```python
from build123d import *
from OCP.BRepFilletAPI import BRepFilletAPI_MakeChamfer

# Parameters (mm, degrees)
SKETCH1_R           = 6.35
BOSS_EXTRUDE1_DEPTH = 450
SKETCH2_W           = 200
SKETCH2_H           = 200
BOSS_EXTRUDE2_DEPTH = 10
CHAMFER1_SIZE       = 10
CHAMFER1_SIZE_2     = 4.663076582
FILLET1_R           = 3


# Some blends are built 0.0001 mm under size
with BuildPart() as part:
    # Sketch1 → Boss-Extrude1 (new body)
    with BuildSketch(Plane(origin=(0, 0, 0), x_dir=(1, 0, 0), z_dir=(0, 1, 0))):
        with Locations(Location((0, 0, 0), (0, 0, 270))):
            Circle(SKETCH1_R)
    extrude(amount=BOSS_EXTRUDE1_DEPTH)

    # Sketch2 → Boss-Extrude2 (add)
    with BuildSketch(Plane(origin=(0, 0, 0), x_dir=(1, 0, 0), z_dir=(0, 1, 0))):
        with Locations((0, -70)):
            Rectangle(SKETCH2_W, SKETCH2_H)
    extrude(amount=BOSS_EXTRUDE2_DEPTH)

    # Chamfer1
    chamfer1_edges_1 = [part.edges().sort_by_distance(p)[0] for p in [
        (-100, 10, 70),
    ]]
    chamfer1_side_1 = [part.faces().sort_by_distance(p)[0] for p in [
        (-100, 9.906738468, 70),
    ]]
    chamfer1_edges_2 = [part.edges().sort_by_distance(p)[0] for p in [
        (0, 10, -30),
    ]]
    chamfer1_side_2 = [part.faces().sort_by_distance(p)[0] for p in [
        (0, 9.906738468, -30),
    ]]
    chamfer1_edges_3 = [part.edges().sort_by_distance(p)[0] for p in [
        (100, 10, 70),
    ]]
    chamfer1_side_3 = [part.faces().sort_by_distance(p)[0] for p in [
        (100, 9.906738468, 70),
    ]]
    chamfer1_edges_4 = [part.edges().sort_by_distance(p)[0] for p in [
        (0, 10, 170),
    ]]
    chamfer1_side_4 = [part.faces().sort_by_distance(p)[0] for p in [
        (0, 9.906738468, 170),
    ]]
    chamfer1 = BRepFilletAPI_MakeChamfer(part.part.solid().wrapped)
    for e in chamfer1_edges_1:
        chamfer1.Add(CHAMFER1_SIZE - 0.0001, CHAMFER1_SIZE_2 - 0.0001, e.wrapped, chamfer1_side_1[0].wrapped)
    for e in chamfer1_edges_2:
        chamfer1.Add(CHAMFER1_SIZE - 0.0001, CHAMFER1_SIZE_2 - 0.0001, e.wrapped, chamfer1_side_2[0].wrapped)
    for e in chamfer1_edges_3:
        chamfer1.Add(CHAMFER1_SIZE - 0.0001, CHAMFER1_SIZE_2 - 0.0001, e.wrapped, chamfer1_side_3[0].wrapped)
    for e in chamfer1_edges_4:
        chamfer1.Add(CHAMFER1_SIZE - 0.0001, CHAMFER1_SIZE_2 - 0.0001, e.wrapped, chamfer1_side_4[0].wrapped)
    add(Compound.cast(chamfer1.Shape()), mode=Mode.REPLACE)  # a hair under: the kernel refuses the full size

    # Fillet1
    # the kernel refuses this fillet: 3 mm, written as the material it takes off along each edge
    with BuildSketch(Plane(origin=(93.425803391, 7, 163.425803391), x_dir=(0.8181037420217215, -0.5211920852493197, 0.24303307915492178), z_dir=(0.40339585418655427, 0.8213060146195212, 0.4033958541865531))) as fillet1_piece_1_section:
        Polygon((-4.845611884, -4.845611884), (4.845611884, -4.845611884), (4.845611884, 4.845611884), (-4.845611884, 4.845611884), align=None)
    fillet1_piece_1 = extrude(amount=4.845611884, mode=Mode.PRIVATE)
    fillet1_piece_1 = split(fillet1_piece_1, bisect_by=Plane(origin=(93.425803391, 7, 163.425803391), z_dir=(-0.3892785155895378, 0.834820025275396, -0.3892785155895367)), keep=Keep.TOP, mode=Mode.PRIVATE)
    fillet1_piece_1 = split(fillet1_piece_1, bisect_by=Plane(origin=(93.425803391, 7, 163.425803391), z_dir=(0, 0, 1)), keep=Keep.TOP, mode=Mode.PRIVATE)
    fillet1_piece_1 = split(fillet1_piece_1, bisect_by=Plane(origin=(93.425803391, 7, 163.425803391), z_dir=(1, 0, 0)), keep=Keep.TOP, mode=Mode.PRIVATE)
    fillet1_piece_1 = split(fillet1_piece_1, bisect_by=Plane(origin=(93.425803391, 8.267842866, 166.14473231), z_dir=(-2.562508249607615e-15, -0.42261428872649237, -0.9063096396729988)), keep=Keep.TOP, mode=Mode.PRIVATE)
    fillet1_piece_1 = split(fillet1_piece_1, bisect_by=Plane(origin=(96.14473231, 8.267842866, 163.425803391), z_dir=(-0.9063096396729988, -0.4226142887264923, 0)), keep=Keep.TOP, mode=Mode.PRIVATE)
    fillet1_piece_1 = split(fillet1_piece_1, bisect_by=Plane(origin=(93.425803391, 10, 163.425803391), z_dir=(0, -1, 0)), keep=Keep.TOP, mode=Mode.PRIVATE)
    fillet1_piece_1 = fillet1_piece_1 - Plane(origin=(93.425803391, 7, 163.425803391), x_dir=(-0.40339585418655427, -0.8213060146195212, -0.4033958541865531), z_dir=(0.8181037420217215, -0.5211920852493197, 0.24303307915492178)) * Sphere(FILLET1_R, mode=Mode.PRIVATE)
    add(fillet1_piece_1, mode=Mode.SUBTRACT)
    with BuildSketch(Plane(origin=(-93.425803391, 7, 163.425803391), x_dir=(-0.24303307915492378, -0.5211920852493191, 0.8181037420217212), z_dir=(-0.4033958541865524, 0.821306014619522, 0.4033958541865535))) as fillet1_piece_2_section:
        Polygon((-4.845611884, -4.845611884), (4.845611884, -4.845611884), (4.845611884, 4.845611884), (-4.845611884, 4.845611884), align=None)
    fillet1_piece_2 = extrude(amount=4.845611884, mode=Mode.PRIVATE)
    fillet1_piece_2 = split(fillet1_piece_2, bisect_by=Plane(origin=(-93.425803391, 7, 163.425803391), z_dir=(0.3892785155895374, 0.8348200252753952, -0.38927851558953863)), keep=Keep.TOP, mode=Mode.PRIVATE)
    fillet1_piece_2 = split(fillet1_piece_2, bisect_by=Plane(origin=(-93.425803391, 7, 163.425803391), z_dir=(-1, 0, 0)), keep=Keep.TOP, mode=Mode.PRIVATE)
    fillet1_piece_2 = split(fillet1_piece_2, bisect_by=Plane(origin=(-93.425803391, 7, 163.425803391), z_dir=(0, 0, 1)), keep=Keep.TOP, mode=Mode.PRIVATE)
    fillet1_piece_2 = split(fillet1_piece_2, bisect_by=Plane(origin=(-96.14473231, 8.267842866, 163.425803391), z_dir=(0.9063096396729988, -0.4226142887264923, 0)), keep=Keep.TOP, mode=Mode.PRIVATE)
    fillet1_piece_2 = split(fillet1_piece_2, bisect_by=Plane(origin=(-93.425803391, 8.267842866, 166.14473231), z_dir=(-2.562508249607615e-15, -0.42261428872649237, -0.9063096396729988)), keep=Keep.TOP, mode=Mode.PRIVATE)
    fillet1_piece_2 = split(fillet1_piece_2, bisect_by=Plane(origin=(-93.425803391, 10, 163.425803391), z_dir=(0, -1, 0)), keep=Keep.TOP, mode=Mode.PRIVATE)
    fillet1_piece_2 = fillet1_piece_2 - Plane(origin=(-93.425803391, 7, 163.425803391), x_dir=(0.4033958541865524, -0.821306014619522, -0.4033958541865535), z_dir=(-0.24303307915492378, -0.5211920852493191, 0.8181037420217212)) * Sphere(FILLET1_R, mode=Mode.PRIVATE)
    add(fillet1_piece_2, mode=Mode.SUBTRACT)
    with BuildSketch(Plane(origin=(93.425803391, 7, -23.425803391), x_dir=(-0.8181037420217211, 0.5211920852493194, 0.2430330791549239), z_dir=(0.4033958541865533, 0.8213060146195218, -0.4033958541865533))) as fillet1_piece_3_section:
        Polygon((-4.845611884, -4.845611884), (4.845611884, -4.845611884), (4.845611884, 4.845611884), (-4.845611884, 4.845611884), align=None)
    fillet1_piece_3 = extrude(amount=4.845611884, mode=Mode.PRIVATE)
    fillet1_piece_3 = split(fillet1_piece_3, bisect_by=Plane(origin=(93.425803391, 7, -23.425803391), z_dir=(-0.3892785155895376, 0.8348200252753957, 0.3892785155895376)), keep=Keep.TOP, mode=Mode.PRIVATE)
    fillet1_piece_3 = split(fillet1_piece_3, bisect_by=Plane(origin=(93.425803391, 7, -23.425803391), z_dir=(0, 0, -1)), keep=Keep.TOP, mode=Mode.PRIVATE)
    fillet1_piece_3 = split(fillet1_piece_3, bisect_by=Plane(origin=(93.425803391, 7, -23.425803391), z_dir=(1, 0, 0)), keep=Keep.TOP, mode=Mode.PRIVATE)
    fillet1_piece_3 = split(fillet1_piece_3, bisect_by=Plane(origin=(93.425803391, 8.267842866, -26.14473231), z_dir=(0, -0.4226142887264923, 0.9063096396729988)), keep=Keep.TOP, mode=Mode.PRIVATE)
    fillet1_piece_3 = split(fillet1_piece_3, bisect_by=Plane(origin=(96.14473231, 8.267842866, -23.425803391), z_dir=(-0.9063096396729988, -0.4226142887264923, 0)), keep=Keep.TOP, mode=Mode.PRIVATE)
    fillet1_piece_3 = split(fillet1_piece_3, bisect_by=Plane(origin=(93.425803391, 10, -23.425803391), z_dir=(0, -1, 0)), keep=Keep.TOP, mode=Mode.PRIVATE)
    fillet1_piece_3 = fillet1_piece_3 - Plane(origin=(93.425803391, 7, -23.425803391), x_dir=(-0.4033958541865533, -0.8213060146195218, 0.4033958541865533), z_dir=(-0.8181037420217211, 0.5211920852493194, 0.2430330791549239)) * Sphere(FILLET1_R, mode=Mode.PRIVATE)
    add(fillet1_piece_3, mode=Mode.SUBTRACT)
    with BuildSketch(Plane(origin=(-93.425803391, 7, -23.425803391), x_dir=(0.2430330791549239, 0.5211920852493194, 0.8181037420217211), z_dir=(-0.4033958541865533, 0.8213060146195218, -0.4033958541865533))) as fillet1_piece_4_section:
        Polygon((-4.845611884, -4.845611884), (4.845611884, -4.845611884), (4.845611884, 4.845611884), (-4.845611884, 4.845611884), align=None)
    fillet1_piece_4 = extrude(amount=4.845611884, mode=Mode.PRIVATE)
    fillet1_piece_4 = split(fillet1_piece_4, bisect_by=Plane(origin=(-93.425803391, 7, -23.425803391), z_dir=(0.3892785155895376, 0.8348200252753957, 0.3892785155895376)), keep=Keep.TOP, mode=Mode.PRIVATE)
    fillet1_piece_4 = split(fillet1_piece_4, bisect_by=Plane(origin=(-93.425803391, 7, -23.425803391), z_dir=(-1, 0, 0)), keep=Keep.TOP, mode=Mode.PRIVATE)
    fillet1_piece_4 = split(fillet1_piece_4, bisect_by=Plane(origin=(-93.425803391, 7, -23.425803391), z_dir=(0, 0, -1)), keep=Keep.TOP, mode=Mode.PRIVATE)
    fillet1_piece_4 = split(fillet1_piece_4, bisect_by=Plane(origin=(-96.14473231, 8.267842866, -23.425803391), z_dir=(0.9063096396729988, -0.4226142887264923, 0)), keep=Keep.TOP, mode=Mode.PRIVATE)
    fillet1_piece_4 = split(fillet1_piece_4, bisect_by=Plane(origin=(-93.425803391, 8.267842866, -26.14473231), z_dir=(0, -0.4226142887264923, 0.9063096396729988)), keep=Keep.TOP, mode=Mode.PRIVATE)
    fillet1_piece_4 = split(fillet1_piece_4, bisect_by=Plane(origin=(-93.425803391, 10, -23.425803391), z_dir=(0, -1, 0)), keep=Keep.TOP, mode=Mode.PRIVATE)
    fillet1_piece_4 = fillet1_piece_4 - Plane(origin=(-93.425803391, 7, -23.425803391), x_dir=(0.4033958541865533, -0.8213060146195218, 0.4033958541865533), z_dir=(0.2430330791549239, 0.5211920852493194, 0.8181037420217211)) * Sphere(FILLET1_R, mode=Mode.PRIVATE)
    add(fillet1_piece_4, mode=Mode.SUBTRACT)
    with BuildSketch(Plane(origin=(93.425803391, 10, 165.337023418), x_dir=(0, -0.9063096396729513, 0.4226142887265943), z_dir=(-1, 0, 0)), Plane(origin=(95.337023418, 10, -23.425803391), x_dir=(0.4226142887264939, -0.9063096396729982, 0), z_dir=(0, 0, 1))) as fillet1_piece_5:
        with BuildLine():
            CenterArc((FILLET1_R * 0.637073342265, -FILLET1_R), FILLET1_R, 90, 65.000251169)
            Line((-FILLET1_R * 0.269236297408, -FILLET1_R * 0.577385711273), (0, 0))
            Line((0, 0), (FILLET1_R * 0.637073342265, 0))
        make_face()
    extrude(amount=186.851606782, mode=Mode.SUBTRACT)
    with BuildSketch(Plane(origin=(-93.425803391, 10, -25.337023418), x_dir=(0, 0, 1), z_dir=(1, 0, 0)), Plane(origin=(-95.337023418, 10, 163.425803391), x_dir=(1, 0, 0), z_dir=(0, 0, -1))) as fillet1_piece_6:
        with BuildLine():
            CenterArc((FILLET1_R * 0.637073342265, FILLET1_R), FILLET1_R, 204.999748831, 65.000251169)
            Line((-FILLET1_R * 0.269236297408, FILLET1_R * 0.577385711274), (0, 0))
            Line((0, 0), (FILLET1_R * 0.637073342265, 0))
        make_face()
    extrude(amount=186.851606782, mode=Mode.SUBTRACT)
    with BuildSketch(Plane(origin=(102.437331252, -5.22683356, -32.437331252), x_dir=(0.16451466298238407, -0.3528068711963904, 0.9211200992815249), z_dir=(-0.3892785155895376, 0.8348200252753957, 0.3892785155895376)), Plane(origin=(102.437331252, -5.22683356, 172.437331252), x_dir=(-0.9211200992815247, -0.3528068711963899, 0.16451466298238568), z_dir=(-0.38927851558953774, 0.834820025275396, -0.3892785155895367))) as fillet1_piece_7:
        with BuildLine():
            CenterArc((FILLET1_R * 0.834820025275, -FILLET1_R), FILLET1_R, 90, 79.711610414)
            Line((-FILLET1_R * 0.149101224928, -FILLET1_R * 0.821397162964), (0, 0))
            Line((0, 0), (FILLET1_R * 0.834820025275, 0))
        make_face()
    extrude(amount=17.223193879, mode=Mode.SUBTRACT)
    with BuildSketch(Plane(origin=(-102.437331252, -5.22683356, -32.437331252), x_dir=(-0.16451466298237352, -0.35280687119639537, 0.9211200992815248), z_dir=(0.3892785155895376, 0.8348200252753957, 0.3892785155895376)), Plane(origin=(-102.437331252, -5.22683356, 172.437331252), x_dir=(0.9211200992815248, -0.35280687119640064, 0.16451466298236184), z_dir=(0.38927851558953747, 0.8348200252753953, -0.38927851558953863))) as fillet1_piece_8:
        with BuildLine():
            CenterArc((FILLET1_R * 0.834820025275, FILLET1_R), FILLET1_R, 190.288389586, 79.711610414)
            Line((-FILLET1_R * 0.149101224928, FILLET1_R * 0.821397162964), (0, 0))
            Line((0, 0), (FILLET1_R * 0.834820025275, 0))
        make_face()
    extrude(amount=17.223193879, mode=Mode.SUBTRACT)


solid = part.part
```
Geometry check sheet. Reference: the model listing, model coordinates, mm. A direction names the side the tool comes from. Coordinates: 2 decimals unless noted, no trailing zeros. Order: outer loops, then holes, each group sorted by start corner. A loop starts at its lowest first (then second) coordinate and runs counter-clockwise, first axis right, second up. Notation, with made-up numbers: (35.25, 78.5) - (45.25, 78.5) arc R21 ccw to (45.25, 107.5) - close; hole circle Ø2 at (3.25, 88). An arc over 180 degrees is marked (long way). Answer in a Markdown table with one row per item. Add a question column.
1. Access from +Z, -Z, +X, -X, +Y, -Y to the whole of each face (thin tool, end or side, straight path). Record for faces 1 (the face through (-3.86, 226.92, -5.04)), 2 (the face through (-1.362, 4.192, -28.045)).
2. Gauge pin test, flat ends, axial feed: pin 1 Ø2 at (x, y) = (-2.5, 116) entering from -Z; pin 2 Ø5 at (y, z) = (248.5, 9) entering from -X. Record the tip position at first contact, or that the pin passes through.
3. Section check D-D (y = 233). Enter the section's corners in (x, z), plus the area to 3 significant figures.
4. Material ranges on L1, parallel to Y at x = 35.5, z = 137; L2, parallel to Z at x = 0, y = 168; L3, parallel to Z at x = -3.5, y = 27, recorded low to high. Write a range as [from, to].
Data:
| question | item | result |
|---|---|---|
| 1 | face 1 | +Y |
| 1 | face 2 | -Z, +X, -X, +Y |
| 2 | pin 1 | stops at z = -6.17 |
| 2 | pin 2 | passes through |
| 3 | outline | circle Ø12.7 at (0, 0) |
| 3 | area | 127 mm² |
| 4 | L1 | y = [0, 10] |
| 4 | L2 | z = [-6.35, 6.35] |
| 4 | L3 | z = [-5.3, 5.3] |
